```python
from build123d import *

# Parameters (mm, degrees)
F0_W     = 42.796455
F0_H     = 26.70499
F1_DEPTH = 25.4
F2_R     = 5.08
F3_SIZE  = 5.08
F4_R     = 6.183466
F5_DEPTH = 25.4


with BuildPart() as f1:
    # F0 (on Front) → F1 (new body)
    with BuildSketch(Plane.XZ):
        with Locations((-113.325018, 16.9474)):
            Rectangle(F0_W, F0_H)
    extrude(amount=F1_DEPTH)

    # F2
    f2_edges = [f1.edges().sort_by_distance(p)[0] for p in [
        (-91.926791, -12.7, 30.299895),
    ]]
    fillet(f2_edges, radius=F2_R)

    # F3
    f3_edges = [f1.edges().sort_by_distance(p)[0] for p in [
        (-115.865018, -25.4, 30.299895),
    ]]
    chamfer(f3_edges, length=F3_SIZE)

    # F4 (on face) → F5 (cut)
    with BuildSketch(Plane(origin=(0, 0, 3.594905), x_dir=(1, 0, 0), z_dir=(0, 0, -1))):
        with Locations((-116.761126, 10.623152)):
            Circle(F4_R)
    extrude(amount=-F5_DEPTH, mode=Mode.SUBTRACT)


solid = f1.part
```
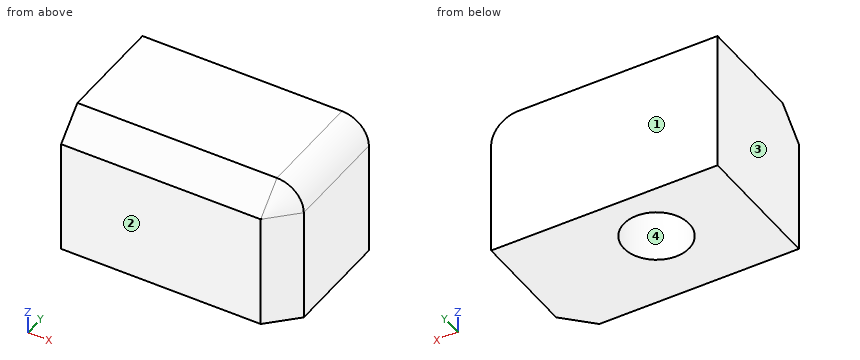
Part model, mm, in its own coordinate system. Face numbers are marked on the shaded views. Coordinates: 2 decimals unless noted, no trailing zeros. Order: outer loops, then holes, each group sorted by start corner. A loop starts at its lowest first (then second) coordinate and runs counter-clockwise, first axis right, second up. Notation, with made-up numbers: (50, 50) - (100, 50) arc R27 cw to (100, 78) - close; hole circle Ø4 at (28, 55). An arc over 180 degrees is marked (long way). Return JSON: item names as keys, results as strings. Group by question number.
Item 1: Pull direction Y, two halves, no side cores. Call the marked faces 1, 2, 3 and 4: pulls with the +Y half, pulls with the -Y half, needs draft (parallel to the pull), parting line crosses it, or undercut.
Item 2: Cut at B-B (x = -121.5). List the corners of the cut face in (y, z).
Item 3: Drill centre lines: probe 1 along X at (y, z) = (-10.75, 13.75); probe 2 along Z at (x, y) = (-115, -10.75); probe 3 along Y at (x, z) = (-122, 12.25). Where is each one in solid material? Low to high. Write a range as from..to.
Item 4: Cut at A-A (z = 12.75). List the corners of the cut face in (x, y).
Item 5: Cut at D-D (x = -129). List the corners of the cut face in (y, z), plus the area to 3 significant figures.
Item 6: Pin check, flat tips, straight feed: pin 1 (2 mm diameter, centred on x = -128.5, y = -22.5, fed in from +Z); pin 2 (11 mm diameter, centred on x = -116.76, y = -10.62, fed in from -Z). Stop position of each tip, or through.
Item 7: Cut at C-C (y = -8.75). List the corners of the cut face in (x, z).
Check values:
{
 "1": {"face 1": "pulls with the +Y half", "face 2": "pulls with the -Y half", "face 3": "needs draft", "face 4": "undercut"},
 "2": {"outline": "(-25.4, 3.59) - (-14.6, 3.59) - (-14.6, 28.99) - (-6.65, 28.99) - (-6.65, 3.59) - (0, 3.59) - (0, 30.3) - (-20.32, 30.3) - (-25.4, 25.22) - close"},
 "3": {"probe 1": "x = -134.72..-122.94, -110.58..-91.93", "probe 2": "z = 28.99..30.3", "probe 3": "y = -25.4..-13.91, -7.34..0"},
 "4": {"outline": "(-134.72, -25.4) - (-97.01, -25.4) - (-91.93, -20.32) - (-91.93, 0) - (-134.72, 0) - close; hole circle Ø12.37 at (-116.76, -10.62)"},
 "5": {"outline": "(-25.4, 3.59) - (0, 3.59) - (0, 30.3) - (-20.32, 30.3) - (-25.4, 25.22) - close", "area": "665 mm2"},
 "6": {"pin 1": "stops at z = 29.12", "pin 2": "stops at z = 28.99"},
 "7": {"outline": "(-134.72, 3.59) - (-122.65, 3.59) - (-122.65, 28.99) - (-110.87, 28.99) - (-110.87, 3.59) - (-91.93, 3.59) - (-91.93, 25.22) arc R5.08 ccw to (-97.01, 30.3) - (-134.72, 30.3) - close"}
}
